Geometry: final body of the model. Coordinates: model frame, mm. A direction names the side the tool comes from. Give positions to 0.01 mm unless a question says otherwise; leave off trailing zeros. Write each loop counter-clockwise with the first axis right and the second up, starting at its lowest first coordinate (ties: lowest second). Pieces come first, ordered by that corner, then holes.
Q1. Cut plane B-B on y = 28. Return the cut outline in (x, z), plus the area to 3 significant figures.
Q2. Cut plane D-D on y = -19.5. Return the cut outline in (x, z), plus the area to 3 significant figures.
Q3. Cut plane A-A on z = 0.35. Count the separate pieces of the cut face and the enclosed holes in it, plus the area to 3 significant figures.
Q4. Line query: L1, parallel to Y at x = 0, z = 0.65; L2, parallel to Y at x = 28, z = 1.3; L3, parallel to X at y = -15, z = 1.65. Output: solid intervals per line, ascending.
Q5. Draft query along Y for faces 1 (the face through (7.71, -7.8, 0.99)), 2 (the face through (-6, -20, 1)), 3 (the face through (-7.493, 0.33, 0.986)). Return one class per face: pulls with the +Y half, pulls with the -Y half, needs draft (parallel to the pull), parting line crosses it, or undercut.
Q6. Pin query (flat end, axial travel): pin 1 (6 mm diameter, centred on x = -0.5, y = 15.5, fed in from +Z); pin 2 (12 mm diameter, centred on x = 0, y = 0, fed in from +Z); pin 3 (0.6 mm diameter, centred on y = -24, z = 0.5, fed in from +X); pin 4 (0.6 mm diameter, centred on x = 19, z = 0.5, fed in from -Y). Return the tip coordinate at first contact, or that it passes through.
Q7. Reachability of faces 4 (the face through (-4.29, -33.2, 0.99)), 5 (the face through (-20, 6, 1)) from +Z, -Z, +X, -X, +Y, -Y: full face, straight path, thin tool, end or side. Return the list, or none.
```python
from build123d import *

# Parameters (mm, degrees)
SKETCH1_R           = 7.5
SKETCH1_R_2         = 2.05
SKETCH1_R_3         = 1.5
BOSS_EXTRUDE1_DEPTH = 2


with BuildPart() as part:
    # Sketch1 → Boss-Extrude1 (new body)
    with BuildSketch(Plane.XY):
        with BuildLine():
            Line((11.99, -6), (29.01, -6))
            ThreePointArc((29.01, -6), (33.245569619, -4.245569619), (35, -0.01))
            Line((35, -0.01), (35, 0.01))
            ThreePointArc((35, 0.01), (33.245569619, 4.245569619), (29.01, 6))
            Line((29.01, 6), (11.99, 6))
            ThreePointArc((11.99, 6), (7.754430381, 7.754430381), (6, 11.99))
            Line((6, 11.99), (6, 29.01))
            ThreePointArc((6, 29.01), (4.245569619, 33.245569619), (0.01, 35))
            Line((0.01, 35), (-0.01, 35))
            ThreePointArc((-0.01, 35), (-4.245569619, 33.245569619), (-6, 29.01))
            Line((-6, 29.01), (-6, 11.99))
            ThreePointArc((-6, 11.99), (-7.754430381, 7.754430381), (-11.99, 6))
            Line((-11.99, 6), (-29.01, 6))
            ThreePointArc((-29.01, 6), (-33.245569619, 4.245569619), (-35, 0.01))
            Line((-35, 0.01), (-35, -0.01))
            ThreePointArc((-35, -0.01), (-33.245569619, -4.245569619), (-29.01, -6))
            Line((-29.01, -6), (-11.99, -6))
            ThreePointArc((-11.99, -6), (-7.754430381, -7.754430381), (-6, -11.99))
            Line((-6, -11.99), (-6, -29.01))
            ThreePointArc((-6, -29.01), (-4.245569619, -33.245569619), (-0.01, -35))
            Line((-0.01, -35), (0.01, -35))
            ThreePointArc((0.01, -35), (4.245569619, -33.245569619), (6, -29.01))
            Line((6, -29.01), (6, -11.99))
            ThreePointArc((6, -11.99), (7.754430381, -7.754430381), (11.99, -6))
        make_face()
        Circle(SKETCH1_R, mode=Mode.SUBTRACT)
        with Locations((-28, 0)):
            Circle(SKETCH1_R_2, mode=Mode.SUBTRACT)
        with Locations(Location((28, 0, 0), (0, 0, 180))):
            Circle(SKETCH1_R_2, mode=Mode.SUBTRACT)
        with Locations((0, 28)):
            Circle(SKETCH1_R_2, mode=Mode.SUBTRACT)
        with Locations(Location((0, -28, 0), (0, 0, 180))):
            Circle(SKETCH1_R_2, mode=Mode.SUBTRACT)
        with Locations((0, 15)):
            Circle(SKETCH1_R_3, mode=Mode.SUBTRACT)
        with Locations(Location((0, -15, 0), (0, 0, 180))):
            Circle(SKETCH1_R_3, mode=Mode.SUBTRACT)
        with Locations((-15, 0)):
            Circle(SKETCH1_R_3, mode=Mode.SUBTRACT)
        with Locations(Location((15, 0, 0), (0, 0, 180))):
            Circle(SKETCH1_R_3, mode=Mode.SUBTRACT)
    extrude(amount=BOSS_EXTRUDE1_DEPTH)


solid = part.part
```
Data:
1. outline: (-6, 0) - (-2.05, 0) - (-2.05, 2) - (-6, 2) - close; (2.05, 0) - (6, 0) - (6, 2) - (2.05, 2) - close
1. area: 15.8 mm2
2. outline: (-6, 0) - (6, 0) - (6, 2) - (-6, 2) - close
2. area: 24.0 mm2
3. separate pieces: 1
3. enclosed holes: 9
3. area: 1,250 mm2
4. L1: y = -35 to -30.05, -25.95 to -16.5, -13.5 to -7.5, 7.5 to 13.5, 16.5 to 25.95, 30.05 to 35
4. L2: y = -6 to -2.05, 2.05 to 6
4. L3: x = -6 to -1.5, 1.5 to 6
5. face 1: pulls with the -Y half
5. face 2: needs draft
5. face 3: undercut
6. pin 1: stops at z = 2
6. pin 2: passes through
6. pin 3: stops at x = 6
6. pin 4: stops at y = -6
7. face 4: +Z, -Z, -X, -Y
7. face 5: +Z, -Z, -X, +Y
